```python
from build123d import *

# Parameters (mm, degrees)
SKETCH1_W           = 12.7
SKETCH1_H           = 12.7
BOSS_EXTRUDE1_DEPTH = 2.54
FILLET1_R           = 0.635
SHELL1_START        = 0.635
SHELL1_OUTLINE_W    = 1.905
SHELL1_OUTLINE_H    = 11.43
SHELL1_DEPTH        = 11.43
SKETCH2_R           = 2.54
BOSS_EXTRUDE2_DEPTH = 1.905
BOSS_EXTRUDE3_DEPTH = 0.00254


# Read off the part's stored shape, not the designer's step: Shell1
with BuildPart() as part:
    # Sketch1 → Boss-Extrude1 (new body)
    with BuildSketch(Plane(origin=(0, 0, 0), x_dir=(1, 0, 0), z_dir=(0, 1, 0))):
        with Locations((6.35, 6.35)):
            Rectangle(SKETCH1_W, SKETCH1_H)
    extrude(amount=BOSS_EXTRUDE1_DEPTH)

    # Fillet1
    fillet1_edges = [part.edges().sort_by_distance(p)[0] for p in [
        (0, 1.27, -12.7),
        (12.7, 1.27, -12.7),
        (12.7, 1.27, 0),
        (0, 1.27, 0),
    ]]
    fillet(fillet1_edges, radius=FILLET1_R)

    # Shell1 outline → Shell1 (cut)
    with BuildSketch(Plane.YZ.offset(SHELL1_START)):
        with Locations((0.9525, -6.35)):
            Rectangle(SHELL1_OUTLINE_W, SHELL1_OUTLINE_H)
    extrude(amount=SHELL1_DEPTH, mode=Mode.SUBTRACT)

    # Sketch2 → Boss-Extrude2 (add)
    with BuildSketch(Plane(origin=(0, 1.905, 0), x_dir=(-1, 0, 0), z_dir=(0, -1, 0))):
        with Locations(Location((-6.35, 6.35, 0), (0, 0, 270))):
            Circle(SKETCH2_R)
    extrude(amount=BOSS_EXTRUDE2_DEPTH)

    # Sketch3 → Boss-Extrude3 (add)
    with BuildSketch(Plane(origin=(0, 2.54, 0), x_dir=(1, 0, 0), z_dir=(0, 1, 0))):
        Polygon((6.042905248, 8.001), (6.571435897, 8.001), (7.853647436, 4.826), (7.244978566, 4.826), (6.998203726, 5.477282051), (5.614865385, 5.477282051), (5.368090545, 4.826), (4.760057692, 4.826), align=None)
        Polygon((6.306852564, 7.149372396), (5.831111378, 6.047153846), (6.78259375, 6.047153846), align=None, mode=Mode.SUBTRACT)
    extrude(amount=BOSS_EXTRUDE3_DEPTH)


solid = part.part
```
The listing builds one solid part. Answer for the finished solid, in the listing's coordinates (mm). Coordinates: 2 decimals unless noted, no trailing zeros. Loops run counter-clockwise (first coordinate to the right, second up) from the corner with the lowest first, then second, coordinate; pieces in that order, holes last. Notation, with made-up numbers: (-19, -25) -> (21, -25) arc R14 ccw to (21, -17) -> close; hole circle Ø8 at (-2, -13). An arc over 180 degrees is marked (long way). Return JSON: item names as keys, results as strings. Group by question number.
(1) Find the intervals of material crossed by probe 1 along Z at (x, y) = (6.5, 1.75) (3 decimals); probe 2 along Z at (x, y) = (12, 1.4) (3 decimals); probe 3 along X at (y, z) = (1.15, -6.25) (3 decimals), in increasing order. Write a range as from..to.
(2) Given pin 1 Ø3 at (x, z) = (11, -8.5) entering from +Y, flat-ended and moving along its own axis, determine where the tip first touches the part or whether it passes through.
(3) A cutting plane is placed at B-B on x = 9.25. Write down the section's boundary in (y, z) (3 decimals).
(4) Determine the mould class of faces 1 (the flat face through (0, 1, -6)), 2 (the flat face through (6, 1, 0)), 3 (the flat face through (12.065, 1, -6)), 4 (the flat face through (6, 1, -0.635)) for opening direction X: released by +X, released by -X, zero draft, split by the parting line, or undercut.
(5) A cutting plane is placed at C-C on z = -11. Write down the section's boundary in (x, y) (3 decimals), and give its area (3 significant figures).
(6) A cutting plane is placed at A-A on y = 0.9. Write down the section's boundary in (x, z) (3 decimals).
The answers:
{
 "1": {"probe 1": "z = -12.7..-12.065, -8.886..-3.814, -0.635..0", "probe 2": "z = -12.7..-12.065, -0.635..0", "probe 3": "x = 0..0.635, 3.812..8.888, 12.065..12.7"},
 "2": {"pin 1": "stops at y = 2.54"},
 "3": {"outline": "(0, -12.7) -> (2.54, -12.7) -> (2.54, 0) -> (0, 0) -> (0, -0.635) -> (1.905, -0.635) -> (1.905, -12.065) -> (0, -12.065) -> close"},
 "4": {"face 1": "released by -X", "face 2": "zero draft", "face 3": "undercut", "face 4": "undercut"},
 "5": {"outline": "(0, 0) -> (0.635, 0) -> (0.635, 1.905) -> (12.065, 1.905) -> (12.065, 0) -> (12.7, 0) -> (12.7, 2.54) -> (0, 2.54) -> close", "area": "10.5 mm^2"},
 "6": {"outline": "(0, -12.065) arc R0.635 ccw to (0.635, -12.7) -> (12.065, -12.7) arc R0.635 ccw to (12.7, -12.065) -> (12.7, -0.635) arc R0.635 ccw to (12.065, 0) -> (0.635, 0) arc R0.635 ccw to (0, -0.635) -> close; circle Ø5.08 at (6.35, -6.35); hole (0.635, -12.065) -> (12.065, -12.065) -> (12.065, -0.635) -> (0.635, -0.635) -> close"}
}
